from build123d import *

# Parameters (mm, degrees)
SKETCH1_W                        = 140
SKETCH1_H                        = 115
BOSS_EXTRUDE1_DEPTH              = 80
SKETCH3_W                        = 126
SKETCH3_H                        = 66
CUT_EXTRUDE1_DEPTH               = 108
M10X1_0_TAPPED_HOLE1_D           = 9
M10X1_0_TAPPED_HOLE1_DEPTH       = 23
M10X1_0_TAPPED_HOLE1_CBORE_D     = 10
M10X1_0_TAPPED_HOLE1_CBORE_DEPTH = 20
M10X1_0_TAPPED_HOLE1_TIP         = 2.703872786
M10X1_0_TAPPED_HOLE2_D           = 9
M10X1_0_TAPPED_HOLE2_DEPTH       = 23
M10X1_0_TAPPED_HOLE2_CBORE_D     = 10
M10X1_0_TAPPED_HOLE2_CBORE_DEPTH = 20
M10X1_0_TAPPED_HOLE2_TIP         = 2.703872786


with BuildPart() as part:
    # Sketch1 → Boss-Extrude1 (new body)
    with BuildSketch(Plane(origin=(0, 0, 0), x_dir=(1, 0, 0), z_dir=(0, 1, 0))):
        with Locations((23.905213361, 33.54681393)):
            Rectangle(SKETCH1_W, SKETCH1_H)
    extrude(amount=BOSS_EXTRUDE1_DEPTH)

    # Sketch3 → Cut-Extrude1 (cut)
    with BuildSketch(Plane(origin=(0, 0, -91.04681393), x_dir=(-1, 0, 0), z_dir=(0, 0, -1))):
        with Locations((-23.905213361, 40)):
            Rectangle(SKETCH3_W, SKETCH3_H)
    extrude(amount=-CUT_EXTRUDE1_DEPTH, mode=Mode.SUBTRACT)

    # M10x1.0 Tapped Hole1
    with Locations(Plane(origin=(0, 80, 0), x_dir=(1, 0, 0), z_dir=(0, 1, 0))):
        with Locations((-21.094786639, 61.04681393), (38.905213361, 61.04681393)):
            CounterBoreHole(M10X1_0_TAPPED_HOLE1_D / 2, M10X1_0_TAPPED_HOLE1_CBORE_D / 2, M10X1_0_TAPPED_HOLE1_CBORE_DEPTH, depth=M10X1_0_TAPPED_HOLE1_DEPTH)
            with Locations((0, 0, -(M10X1_0_TAPPED_HOLE1_DEPTH + M10X1_0_TAPPED_HOLE1_TIP / 2))):  # 118° drill point
                Cone(0, M10X1_0_TAPPED_HOLE1_D / 2, M10X1_0_TAPPED_HOLE1_TIP, mode=Mode.SUBTRACT)

    # M10x1.0 Tapped Hole2
    with Locations(Plane.ZY.offset(46.094786639)):
        with Locations((-51.04681393, 15)):
            CounterBoreHole(M10X1_0_TAPPED_HOLE2_D / 2, M10X1_0_TAPPED_HOLE2_CBORE_D / 2, M10X1_0_TAPPED_HOLE2_CBORE_DEPTH, depth=M10X1_0_TAPPED_HOLE2_DEPTH)
            with Locations((0, 0, -(M10X1_0_TAPPED_HOLE2_DEPTH + M10X1_0_TAPPED_HOLE2_TIP / 2))):  # 118° drill point
                Cone(0, M10X1_0_TAPPED_HOLE2_D / 2, M10X1_0_TAPPED_HOLE2_TIP, mode=Mode.SUBTRACT)


solid = part.part
For this review, take the finished solid that the model builds, in its own axes (mm). A direction names the side the tool comes from. Coordinates: 2 decimals unless noted, no trailing zeros. Write each loop counter-clockwise with the first axis right and the second up, starting at its lowest first coordinate (ties: lowest second). Pieces come first, ordered by that corner, then holes. Notation, with made-up numbers: (37.25, 69) -> (79.25, 69) arc R19 cw to (79.25, 85) -> close; hole circle Ø7 at (-22.75, 12.25). An arc over 180 degrees is marked (long way). Write each question's results on one line, items separated by ' | '. Start each with the question number.
1) Consider section B-B (y = 15). Write out the cut boundary in (x, z), plus the area to 3 significant figures.
2) Consider section C-C (x = 83). Write out the cut boundary in (y, z).
3) Wall thickness on L1, parallel to Y at x = 11, z = -62.5; L2, parallel to X at y = 22, z = -68.5; L3, parallel to Z at x = -30, y = 27.5: over which ranges is each line inside the solid? List them lowest first. Write a range as [from, to].
4) Insertion check: pin 1 (6 mm diameter, centred on x = 38.91, z = -61.05, fed in from +Y); pin 2 (1 mm diameter, centred on x = 46, y = 14, fed in from -Z); pin 3 (8 mm diameter, centred on y = 15, z = -51.05, fed in from -X). Each pin has a flat end and moves straight along its axis. Give the tip position at first contact, or say it passes through.
5) For faces 4 (the face through (25, 7, -38)), 5 (the face through (35.22, 76.549, -64.426)), 6 (the face through (18, 75, -91.047)), list the 3-axis set-ups (+Z, -Z, +X, -X, +Y, -Y) from which the entire face can be reached by the end or side of a thin tool; tool diameter is ignored.
6) Consider section A-A (z = -42). Write out the cut boundary in (x, y).
7) Consider section D-D (y = 34). Write out the cut boundary in (x, z), plus the area to 3 significant figures.
8) The part is to be moulded in two halves that separate along X. For faces 1 (the face through (-46.095, 39, -33)), 2 (the face through (-39.095, 40, -38)), 3 (the face through (-42.64, 10.12, -52.13)), say which applies: +X half, -X half, draft (parallel to the pull), parting line (faces both ways), or undercut.
Geometry says:
1) outline: (-46.09, -91.05) -> (-39.09, -91.05) -> (-39.09, -56.05) -> (-46.09, -56.05) -> close; (-46.09, -46.05) -> (-39.09, -46.05) -> (-39.09, 16.95) -> (86.91, 16.95) -> (86.91, -91.05) -> (93.91, -91.05) -> (93.91, 23.95) -> (-46.09, 23.95) -> close | area: 2,420 mm^2
2) outline: (0, -91.05) -> (7, -91.05) -> (7, 16.95) -> (73, 16.95) -> (73, -91.05) -> (80, -91.05) -> (80, 23.95) -> (0, 23.95) -> close
3) L1: [0, 7], [73, 80] | L2: [-46.09, -39.09], [86.91, 93.91] | L3: [16.95, 23.95]
4) pin 1: y = 7 | pin 2: z = 16.95 | pin 3: x = 86.91
5) face 4: -Z | face 5: +Y | face 6: -Z, +X, -X, +Y, -Y
6) outline: (-46.09, 0) -> (93.91, 0) -> (93.91, 80) -> (-46.09, 80) -> close; hole (-39.09, 7) -> (86.91, 7) -> (86.91, 73) -> (-39.09, 73) -> close
7) outline: (-46.09, -91.05) -> (-39.09, -91.05) -> (-39.09, 16.95) -> (86.91, 16.95) -> (86.91, -91.05) -> (93.91, -91.05) -> (93.91, 23.95) -> (-46.09, 23.95) -> close | area: 2,490 mm^2
8) face 1: -X half | face 2: undercut | face 3: draft
